Part model, mm, in its own coordinate system. Face numbers are marked on the shaded views. A direction names the side the tool comes from. Coordinates: 2 decimals unless noted, no trailing zeros. Write each loop counter-clockwise with the first axis right and the second up, starting at its lowest first coordinate (ties: lowest second). Pieces come first, ordered by that corner, then holes. Notation, with made-up numbers: M 65,82 L 81,82 A18 cw 81,100 Z; hole C -29.75,83.5 d2. An arc over 180 degrees is marked long. Use a Markdown table: item, result. Add a question column.
Q1. Pin check, flat tips, straight feed: pin 1 Ø1.5 at (x, y) = (-6.5, 6.5) entering from +Z; pin 2 Ø5 at (x, z) = (-6.5, 5) entering from -Y; pin 3 Ø5 at (x, y) = (-5, 2) entering from +Z; pin 4 Ø6 at (y, z) = (7.5, 6.5) entering from -X. Stop position of each tip, or through.
Q2. Mould opens along Y. For the marked faces 1, 2 and 3 say: released by +Y, released by -Y, zero draft, split by the parting line, or undercut.
Q3. Slice it at B-B on y = 5.75. Write the cut outline in (x, z).
Q4. Slice it at A-A on x = -10.25. Write the cut outline in (y, z).
Q5. Wall check: L1, parallel to Z at x = -6.75, y = 9.5; L2, parallel to Z at x = -7.5, y = 5.25; L3, parallel to Y at x = -10, z = 4.75. Give the ranges that are in metal, low to high. Write a range as from..to.
Q6. Tool access for the marked faces 4 and 5: list every direction of +Z, -Z, +X, -X, +Y, -Y with a clear straight run to the whole face (end or side of a thin tool).
Q7. Slice it at D-D on x = -9. Write the cut outline in (y, z), then the cut area to 3 significant figures.
Q8. Slice it at C-C on z = 6.25. Write the cut outline in (x, y).
from build123d import *

# Parameters (mm, degrees)
F0_W     = 12
F0_H     = 1.4
F1_DEPTH = 12
F0_H_2   = 11.6
F0_W_2   = 6.8
F0_H_3   = 3
F2_DEPTH = 1.6
F3_DEPTH = 2.6
F4_W     = 12
F4_H     = 4
F5_DEPTH = 0.6


with BuildPart() as f1:
    # F0 (on Top) → F1 (new body)
    with BuildSketch(Plane.XY):
        with Locations((-6, 12.3)):
            Rectangle(F0_W, F0_H)
    extrude(amount=F1_DEPTH)

    # F0 (on Top) → F2 (join)
    with BuildSketch(Plane.XY):
        with Locations((-6, 5.8)):
            Rectangle(F0_W, F0_H_2)
        with Locations((-6, 6.5)):
            Rectangle(F0_W_2, F0_H_3, mode=Mode.SUBTRACT)
    extrude(amount=F2_DEPTH)

    # F0 (on Top) → F3 (join)
    with BuildSketch(Plane.XY):
        with Locations((-6, 6.5)):
            Rectangle(F0_W_2, F0_H_3)
    extrude(amount=F3_DEPTH)

    # F4 (on face) → F5 (cut)
    with BuildSketch(Plane.XZ.offset(-11.6)):
        with Locations((-6, 10)):
            Rectangle(F4_W, F4_H)
    extrude(amount=-F5_DEPTH, mode=Mode.SUBTRACT)


solid = f1.part
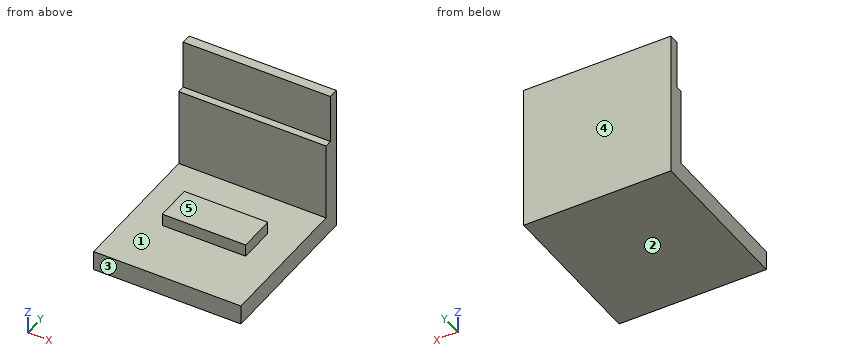
Recorded:
| question | item | result |
|---|---|---|
| 1 | pin 1 | z = 2.6 |
| 1 | pin 2 | y = 5 |
| 1 | pin 3 | z = 1.6 |
| 1 | pin 4 | through |
| 2 | face 1 | undercut |
| 2 | face 2 | zero draft |
| 2 | face 3 | released by -Y |
| 3 | outline | M -12,0 L 0,0 L 0,1.6 L -2.6,1.6 L -2.6,2.6 L -9.4,2.6 L -9.4,1.6 L -12,1.6 Z |
| 4 | outline | M 0,0 L 13,0 L 13,12 L 12.2,12 L 12.2,8 L 11.6,8 L 11.6,1.6 L 0,1.6 Z |
| 5 | L1 | 0..1.6 |
| 5 | L2 | 0..2.6 |
| 5 | L3 | 11.6..13 |
| 6 | face 4 | +Z, -Z, +X, -X, +Y |
| 6 | face 5 | +Z, +X, -X, -Y |
| 7 | outline | M 0,0 L 13,0 L 13,12 L 12.2,12 L 12.2,8 L 11.6,8 L 11.6,1.6 L 8,1.6 L 8,2.6 L 5,2.6 L 5,1.6 L 0,1.6 Z |
| 7 | area | 36.0 mm² |
| 8 | outline | M -12,11.6 L 0,11.6 L 0,13 L -12,13 Z |
